Read the model definition and answer for the solid it produces. Units are mm, in the model's axes. Face numbers are marked on the shaded views. Coordinates: 2 decimals unless noted, no trailing zeros. Loops run counter-clockwise (first coordinate to the right, second up) from the corner with the lowest first, then second, coordinate; pieces in that order, holes last. Notation, with made-up numbers: M 15.25,-24.5 L 68.25,-24.5 A26 cw 68.25,14.5 Z; hole C 18,28 d10. An arc over 180 degrees is marked long. Put each result on its own line as item: value.
from build123d import *

# Parameters (mm, degrees)
BOSS_EXTRUDE1_DEPTH = 4.7
TAP1_D              = 4.134


with BuildPart() as part:
    # Sketch1 → Boss-Extrude1 (new body)
    with BuildSketch(Plane(origin=(0, 0, 0), x_dir=(0, 0, -1), z_dir=(1, 0, 0))):
        Polygon((0, 4.618802154), (-4, 2.309401077), (-4, -2.309401077), (0, -4.618802154), (4, -2.309401077), (4, 2.309401077), align=None)
    extrude(amount=-BOSS_EXTRUDE1_DEPTH)

    # Sketch2 → Cut-Revolve1 (revolve, cut)
    with BuildSketch(Plane.XY):
        Polygon((0, 4), (-0.35726559, 4.618802154), (0, 4.618802154), align=None)
    revolve(axis=Axis((-0.35726559, 0, 0), (1, 0, 0)), mode=Mode.SUBTRACT)

    # Tap1 (through all)
    with Locations(Plane(origin=(0, 0, 0), x_dir=(0, 0, -1), z_dir=(1, 0, 0))):
        with Locations((0, 0)):
            Hole(TAP1_D / 2)


solid = part.part
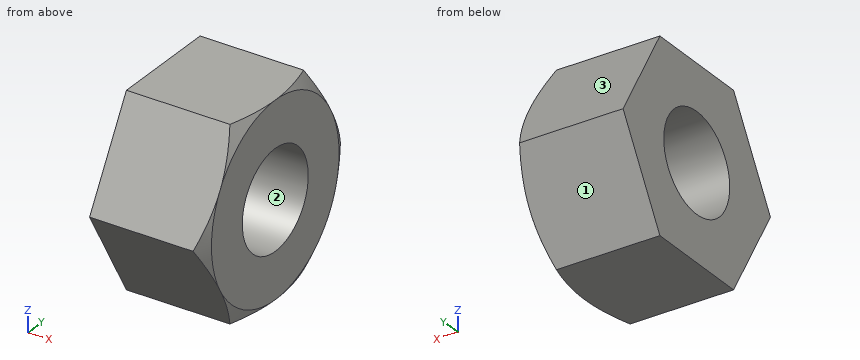
1) Determine the mould class of the marked faces 1, 2 and 3 for opening direction Z: released by +Z, released by -Z, zero draft, split by the parting line, or undercut.
Answer list:
face 1: released by -Z
face 2: undercut
face 3: released by +Z
2) Given pin 1 Ø2.5 at (y, z) = (0, 0) entering from +X; pin 2 Ø1.5 at (x, z) = (-3.5, 2) entering from +Y, each flat-ended and moving along its own axis, determine where each tip first touches the part or whether it passes through.
Answer list:
pin 1: passes through
pin 2: stops at y = 3.9
3) Find section A-A, the plane x = -3.8. Write down the section's boundary in (y, z).
Answer list:
outline: M -4.62,0 L -2.31,-4 L 2.31,-4 L 4.62,0 L 2.31,4 L -2.31,4 Z; hole C 0,0 d4.13
4) Straight lines are drawn through the part: line 1 (Z direction, x = -2.4, y = -2.5); line 2 (Z direction, x = -3.7, y = 0.25); line 3 (Y direction, x = -1.2, z = 3.5). For each, find the intervals that lie inside material, in ascending order. Write a range as [from, to].
Answer list:
line 1: z = [-3.67, 3.67]
line 2: z = [-4, -2.05], [2.05, 4]
line 3: y = [-2.6, 2.6]
